Verification items for the finished model (mm, model axes). Give positions to 0.01 mm unless a question says otherwise; leave off trailing zeros. Loops run counter-clockwise (first coordinate to the right, second up) from the corner with the lowest first, then second, coordinate; pieces in that order, holes last. Notation, with made-up numbers: (18.5, 68.5) - (72.5, 68.5) arc R28 cw to (72.5, 86.5) - close; hole circle Ø5 at (70, -2.5). An arc over 180 degrees is marked (long way). One line per item, written item: value. Start each with the question number.
1. Scan lines: L1, parallel to X at y = 1.75, z = -20; L2, parallel to Z at x = -17.5, y = 0.3; L3, parallel to Z at x = 17, y = 1.25. Record each from-to range of solid material in increasing order. Write a range as [from, to].
2. Sectioned sample at D-D (x = 22). Record the cut outline in (y, z), plus the area to 3 significant figures.
3. Sectioned sample at B-B (y = 1.8). Count the separate pieces of the cut face and the enclosed holes in it, plus the area to 3 significant figures.
4. Sectioned sample at A-A (x = 0). Record the cut outline in (y, z), plus the area to 3 significant figures.
5. Sectioned sample at C-C (z = -15). Record the cut outline in (x, y).
6. Gauge pin test, flat end, axial feed: pin 1 (4 mm diameter, centred on x = 17, z = -20, fed in from -Y). Record the tip position at first contact, or that the pin passes through.
from build123d import *

# Parameters (mm, degrees)
SKETCH1_R                 = 37.5
SKETCH1_R_2               = 6
BOSS_EXTRUDE1_DEPTH       = 4.7625
F_3_0MM_DOWEL_HOLE1_D     = 3
F_3_0MM_DOWEL_HOLE4_D     = 3
F_3_0MM_DOWEL_HOLE4_DEPTH = 10
F_3_0MM_DOWEL_HOLE4_TIP   = 0.901290929


with BuildPart() as part:
    # Sketch1 → Boss-Extrude1 (new body)
    with BuildSketch(Plane(origin=(0, 0, 0), x_dir=(1, 0, 0), z_dir=(0, 1, 0))):
        with Locations(Location((0, 0, 0), (0, 0, 90))):
            Circle(SKETCH1_R)
        with Locations(Location((0, 0, 0), (0, 0, 90))):
            Circle(SKETCH1_R_2, mode=Mode.SUBTRACT)
    extrude(amount=BOSS_EXTRUDE1_DEPTH)

    # Ø3.0mm Dowel Hole1 (through all)
    with Locations(Plane(origin=(0, 0, 0), x_dir=(-1, 0, 0), z_dir=(0, -1, 0))):
        with Locations((0, 15), (0, 22), (22, 0), (15, 0), (0, -15), (0, -22), (-15, 0), (-22, 0)):
            Hole(F_3_0MM_DOWEL_HOLE1_D / 2)

    # Ø3.0mm Dowel Hole4
    with Locations(Plane(origin=(0, 4.7625, 0), x_dir=(1, 0, 0), z_dir=(0, 1, 0))):
        with Locations((-17, 20), (17, -20), (-17, -20), (17, 20)):
            Hole(F_3_0MM_DOWEL_HOLE4_D / 2, depth=F_3_0MM_DOWEL_HOLE4_DEPTH)
            with Locations((0, 0, -(F_3_0MM_DOWEL_HOLE4_DEPTH + F_3_0MM_DOWEL_HOLE4_TIP / 2))):  # 118° drill point
                Cone(0, F_3_0MM_DOWEL_HOLE4_D / 2, F_3_0MM_DOWEL_HOLE4_TIP, mode=Mode.SUBTRACT)


solid = part.part
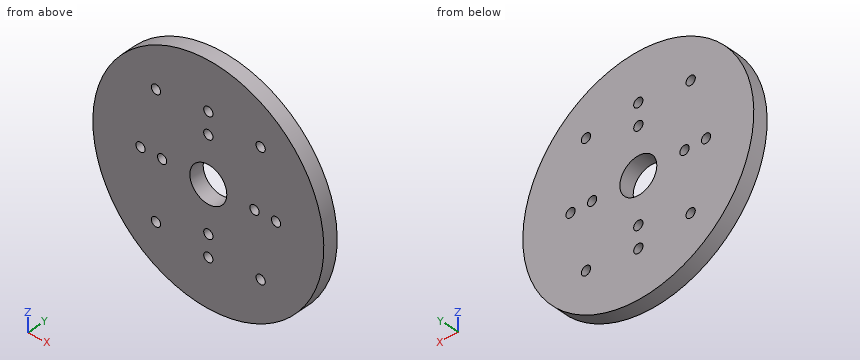
Results are:
1. L1: x = [-31.72, -18.5], [-15.5, 15.5], [18.5, 31.72]
1. L2: z = [-33.17, -21.41], [-18.59, 18.59], [21.41, 33.17]
1. L3: z = [-33.43, -21.5], [-18.5, 18.5], [21.5, 33.43]
2. outline: (0, -30.37) - (4.76, -30.37) - (4.76, -1.5) - (0, -1.5) - close; (0, 1.5) - (4.76, 1.5) - (4.76, 30.37) - (0, 30.37) - close
2. area: 275 mm^2
3. separate pieces: 1
3. enclosed holes: 13
3. area: 4,220 mm^2
4. outline: (0, -37.5) - (4.76, -37.5) - (4.76, -23.5) - (0, -23.5) - close; (0, -20.5) - (4.76, -20.5) - (4.76, -16.5) - (0, -16.5) - close; (0, -13.5) - (4.76, -13.5) - (4.76, -6) - (0, -6) - close; (0, 6) - (4.76, 6) - (4.76, 13.5) - (0, 13.5) - close; (0, 16.5) - (4.76, 16.5) - (4.76, 20.5) - (0, 20.5) - close; (0, 23.5) - (4.76, 23.5) - (4.76, 37.5) - (0, 37.5) - close
4. area: 243 mm^2
5. outline: (-34.37, 0) - (-1.5, 0) - (-1.5, 4.76) - (-34.37, 4.76) - close; (1.5, 0) - (34.37, 0) - (34.37, 4.76) - (1.5, 4.76) - close
6. pin 1: stops at y = 0
